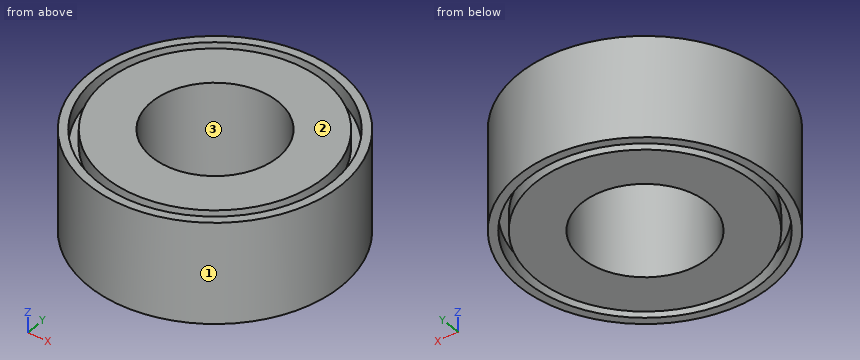
Solid Edge part; units mm, degrees
sketch "Sketch1" plane through (0, 0, 0) normal (0, 0, 1) x (1, 0, 0)
  circle A0 centre (23.6469, 21.2896) radius 15
  circle A1 centre (23.6469, 21.2896) radius 7.5
extrude "ExtrudedProtrusion_1" add sketch "Sketch1" along normal blind 12
sketch "Sketch2" plane through (23.6469, 21.2896, 12) normal (0, 0, 1) x (0, 1, 0)
  circle A0 centre (0, 0) radius 14
  circle A1 centre (0, 0) radius 13
extrude "ExtrudedCutout_1" cut sketch "Sketch2" against normal blind 2
sketch "Sketch3" plane through (23.6469, 21.2896, 0) normal (0, 0, -1) x (0, 1, 0)
  circle A0 centre (0, 0) radius 14
  circle A1 centre (0, 0) radius 13
extrude "ExtrudedCutout_2" cut sketch "Sketch3" against normal blind 2
Can you work these out from the model? Positions are in its coordinate system, mm. Face numbers are marked on the shaded views. Give positions to 0.01 mm unless a question says otherwise; leave off trailing zeros. Order: outer loops, then holes, each group sorted by start corner. A loop starts at its lowest first (then second) coordinate and runs counter-clockwise, first axis right, second up. Notation, with made-up numbers: M 55.25,-9 L 94.25,-9 A33 ccw 94.25,19 Z; hole C 74,14.5 d11. An arc over 180 degrees is marked long. One line per question, with ' | ' between items.
Item 1: Suppose I cut it at A-A, the plane x = 24.5. Write out the boundary of the cut face in (y, z).
Answer block:
outline: M 6.31,0 L 7.32,0 L 7.32,2 L 8.32,2 L 8.32,0 L 13.84,0 L 13.84,12 L 8.32,12 L 8.32,10 L 7.32,10 L 7.32,12 L 6.31,12 Z; M 28.74,0 L 34.26,0 L 34.26,2 L 35.26,2 L 35.26,0 L 36.27,0 L 36.27,12 L 35.26,12 L 35.26,10 L 34.26,10 L 34.26,12 L 28.74,12 Z
Item 2: Suppose I cut it at B-B, the plane y = 21.75. Write out the boundary of the cut face in (x, z), then the cut area to 3 significant figures.
Answer block:
outline: M 8.65,0 L 9.65,0 L 9.65,2 L 10.66,2 L 10.66,0 L 16.16,0 L 16.16,12 L 10.66,12 L 10.66,10 L 9.65,10 L 9.65,12 L 8.65,12 Z; M 31.13,0 L 36.64,0 L 36.64,2 L 37.64,2 L 37.64,0 L 38.64,0 L 38.64,12 L 37.64,12 L 37.64,10 L 36.64,10 L 36.64,12 L 31.13,12 Z | area: 172 mm2
Item 3: Suppose I cut it at C-C, the plane y = 9.25. Write out the boundary of the cut face in (x, z), then the cut area to 3 significant figures.
Answer block:
outline: M 14.7,0 L 16.5,0 L 16.5,2 L 18.74,2 L 18.74,0 L 28.55,0 L 28.55,2 L 30.79,2 L 30.79,0 L 32.59,0 L 32.59,12 L 30.79,12 L 30.79,10 L 28.55,10 L 28.55,12 L 18.74,12 L 18.74,10 L 16.5,10 L 16.5,12 L 14.7,12 Z | area: 197 mm2
Item 4: Suppose I cut it at D-D, the plane x = 15.5. Write out the boundary of the cut face in (y, z), then the cut area to 3 significant figures.
Answer block:
outline: M 8.69,0 L 9.9,0 L 9.9,2 L 11.16,2 L 11.16,0 L 31.42,0 L 31.42,2 L 32.68,2 L 32.68,0 L 33.88,0 L 33.88,12 L 32.68,12 L 32.68,10 L 31.42,10 L 31.42,12 L 11.16,12 L 11.16,10 L 9.9,10 L 9.9,12 L 8.69,12 Z | area: 292 mm2
Item 5: Please list where these lines run through material, in increasing order: L1, parallel to X at y = 21.5, z = 6; L2, parallel to X at y = 27.75, z = 1.25; L3, parallel to Y at x = 19, z = 11.5.
Answer block:
L1: x = 8.65 to 16.15, 31.14 to 38.65 | L2: x = 10.11 to 11.23, 12.37 to 19.84, 27.46 to 34.93, 36.07 to 37.18 | L3: y = 7.03 to 8.08, 9.15 to 15.4, 27.18 to 33.43, 34.5 to 35.55
Item 6: I'm going to push flat-ended pins straight in: pin 1 Ø4 at (x, z) = (15, 4) entering from -Y; pin 2 Ø2 at (y, z) = (10, 10) entering from -X; pin 3 Ø3 at (y, z) = (30.5, 5) entering from -X. Where does each tip first touch, or does it pass through?
Answer block:
pin 1: stops at y = 7.84 | pin 2: stops at x = 12.73 | pin 3: stops at x = 10.78
Item 7: We'd pull the mould along Y, two halves only. Please class the marked faces 1, 2 and 3: released by +Y, released by -Y, zero draft, split by the parting line, or undercut.
Answer block:
face 1: split by the parting line | face 2: zero draft | face 3: undercut
